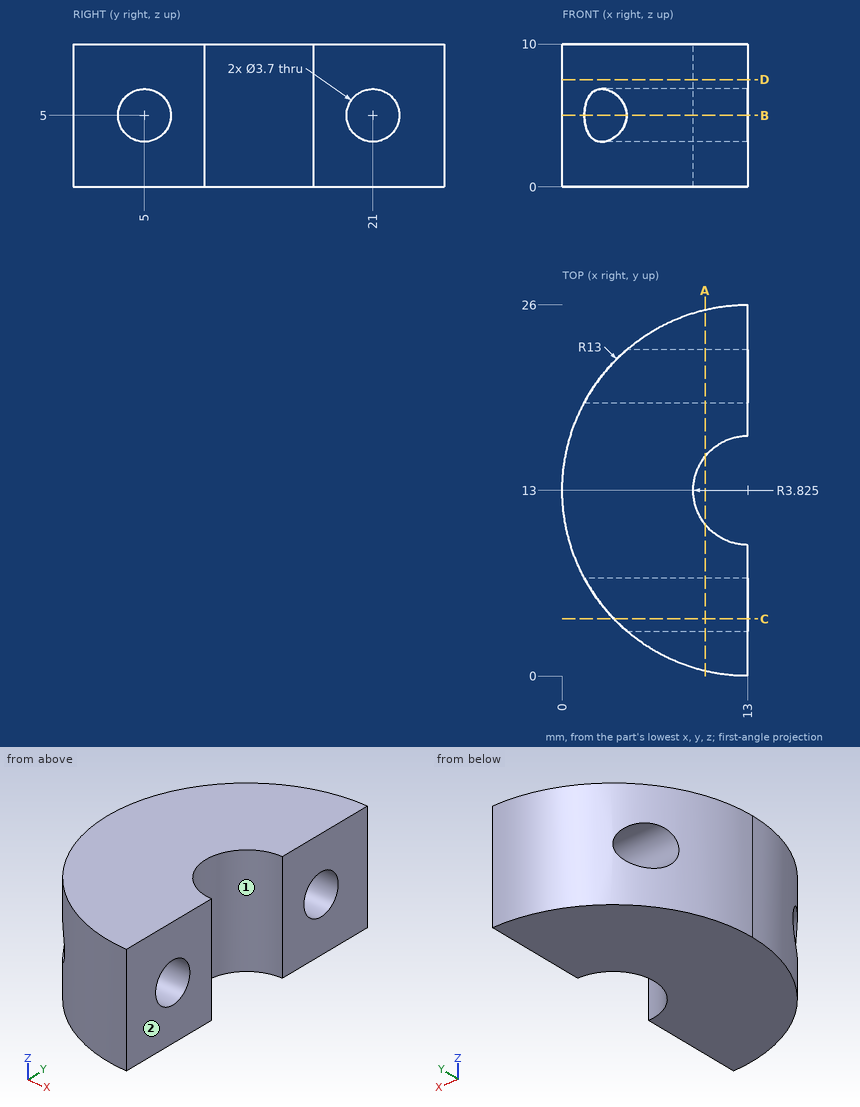
The drawing under review shows one solid part. Ordinate dimensions are in mm from its lowest x, y, z. Round coordinates to 2 decimals unless told otherwise and drop trailing zeros. Loops run counter-clockwise (first coordinate to the right, second up) from the corner with the lowest first, then second, coordinate; pieces in that order, holes last. Notation, with made-up numbers: (-30.5, 17.5) -> (2.5, 17.5) arc R23 cw to (2.5, 37.5) -> close; hole circle Ø8 at (-16, 46). An arc over 180 degrees is marked (long way). One line per question, with ' | ' between items. Start each with the question number.
Item 1: Add section C-C, the plane y = 4. Write out the cut boundary in (x, z).
Item 2: Draft analysis for pull direction Y (two halves, no side actions). For the marked faces 1 and 2, state which applies: +Y half, -Y half, draft (parallel to the pull), parting line (faces both ways), or undercut.
Item 3: Wall thickness on line 1 along Z through (x, y) = (10.25, 21); line 2 along Y through (x, z) = (9, 4); line 3 along Y through (x, z) = (10.5, 0.5): over which ranges is each line inside the solid? List them lowest first. Write a range as [from, to].
Item 4: Add section D-D, the plane z = 7.5. Write out the cut boundary in (x, y) (3 decimals).
Item 5: For pin 1 (6 mm diameter, centred on x = 6.5, z = 3, fed in from -Y); pin 2 (1 mm diameter, centred on x = 11, z = 6.5, fed in from -Y); pin 3 (1 mm diameter, centred on x = 11, z = 5, fed in from +Y), all flat-tipped, find the tip position at first contact; note any pin that passes through.
Item 6: Add section B-B, the plane z = 5. Write out the cut boundary in (x, y) (3 decimals), then the cut area to 3 significant figures.
Item 7: Add section A-A, the plane x = 10. Write out the cut boundary in (y, z), then the cut area to 3 significant figures.
Return value:
1) outline: (3.62, 0) -> (13, 0) -> (13, 3.44) -> (3.62, 3.44) -> close; (3.62, 6.56) -> (13, 6.56) -> (13, 10) -> (3.62, 10) -> close
2) face 1: undercut | face 2: draft
3) line 1: z = [0, 3.15], [6.85, 10] | line 2: y = [0.63, 3.44], [6.56, 19.44], [22.56, 25.37] | line 3: y = [0.24, 10.11], [15.89, 25.76]
4) outline: (13, 0) -> (13, 9.175) arc R3.825 cw to (13, 16.825) -> (13, 26) arc R13 ccw to start
5) pin 1: stops at y = 0.48 | pin 2: stops at y = 0.09 | pin 3: stops at y = 25.91
6) outline: (1.547, 6.85) -> (13, 6.85) -> (13, 9.175) arc R3.825 cw to (13, 16.825) -> (13, 19.15) -> (1.547, 19.15) arc R13 ccw to start; (4.516, 3.15) arc R13 ccw to (13, 0) -> (13, 3.15) -> close; (4.516, 22.85) -> (13, 22.85) -> (13, 26) arc R13 ccw to start | area: 167 mm2
7) outline: (0.35, 0) -> (10.63, 0) -> (10.63, 10) -> (0.35, 10) -> close; (15.37, 0) -> (25.65, 0) -> (25.65, 10) -> (15.37, 10) -> close; hole circle Ø3.7 at (5, 5); hole circle Ø3.7 at (21, 5) | area: 184 mm2
